Design review of the part built by this model. Coordinates are the model's own, in mm. A direction names the side the tool comes from. Coordinates: 2 decimals unless noted, no trailing zeros. Write each loop counter-clockwise with the first axis right and the second up, starting at its lowest first coordinate (ties: lowest second). Pieces come first, ordered by that corner, then holes.
Q1. Add section D-D, the plane z = -4.5. Give the boundary of the cut face in (x, y), plus the area to 3 significant figures.
Q2. Add section C-C, the plane y = 14. Give the boundary of the cut face in (x, z).
Q3. The part is to be moulded in two halves that separate along Y. For faces 1 (the face through (-3.905, 35.586, -0.867)), 2 (the face through (0, 36.6, 0)), 3 (the face through (0, 0, 0)), 4 (the face through (-1.141, 34.206, 3.625)), say which applies: +Y half, -Y half, draft (parallel to the pull), parting line (faces both ways), or undercut.
Q4. Machinability: for faces 5 (the face through (-4.88, 0.99, -1.08)), 6 (the face through (-3.905, 17.677, -0.867)), which of the approach directions +Z, -Z, +X, -X, +Y, -Y give a long, thin tool a straight path to every point of the face, cutting with its end or side? Answer none if there is none.
Q5. Clearance check with flat-ended pins moving along their axes: pin 1 Ø4 at (y, z) = (9.5, -4) entering from -X; pin 2 Ø2 at (x, y) = (-3.5, 32.5) entering from -Z; pin 3 Ø4 at (y, z) = (31, 0) entering from +X. State where each tip first meets the part, or that it passes through.
Q6. To check wall thickness, follow probe 1 along Y at (x, z) = (-2.75, -2.75); probe 2 along Y at (x, z) = (4, -2.25); probe 3 along X at (y, z) = (21, -0.25). State the ranges of each line that lie inside material, in increasing order.
Q7. Add section B-B, the plane x = 0. Give the boundary of the cut face in (y, z).
Q8. Add section A-A, the plane z = 0. Give the boundary of the cut face in (x, y), plus the area to 3 significant figures.
from build123d import *

# Parameters (mm, degrees)
SKETCH_1_R      = 5
EXTRUDE_1_DEPTH = 2
SKETCH_2_R      = 4
EXTRUDE_2_DEPTH = 34.6
SKETCH_3_W      = 0.4
SKETCH_3_H      = 0.8


with BuildPart() as part:
    # 草图1 → 凸台-拉伸1 (new body)
    with BuildSketch(Plane(origin=(0, 0, 0), x_dir=(1, 0, 0), z_dir=(0, 1, 0))):
        with Locations(Location((0, 0, 0), (0, 0, 270))):
            Circle(SKETCH_1_R)
    extrude(amount=EXTRUDE_1_DEPTH)

    # 草图2 → 凸台-拉伸2 (add)
    with BuildSketch(Plane(origin=(0, 2, 0), x_dir=(1, 0, 0), z_dir=(0, 1, 0))):
        with Locations(Location((0, 0, 0), (0, 0, 270))):
            Circle(SKETCH_2_R)
    extrude(amount=EXTRUDE_2_DEPTH)

    # 草图3 → 切除-旋转1 (revolve, cut)
    with BuildSketch(Plane.XY, mode=Mode.PRIVATE) as cut_revolve_1_sk:
        with Locations((4, 34.2)):
            Rectangle(SKETCH_3_W, SKETCH_3_H)
    revolve(cut_revolve_1_sk.sketch.rotate(Axis((0, 36.6, 0), (0, -1, 0)), 90), axis=Axis((0, 36.6, 0), (0, -1, 0)), mode=Mode.SUBTRACT)


solid = part.part
Here are the results:
1. outline: (-2.18, 0) - (2.18, 0) - (2.18, 2) - (-2.18, 2) - close
1. area: 8.72 mm2
2. outline: circle Ø8 at (0, 0)
3. face 1: draft
3. face 2: +Y half
3. face 3: -Y half
3. face 4: undercut
4. face 5: +Y, -Y
4. face 6: +Y
5. pin 1: stops at x = -3.46
5. pin 2: stops at z = -3.12
5. pin 3: stops at x = 4
6. probe 1: y = 0 to 33.8, 34.6 to 36.6
6. probe 2: y = 0 to 2
6. probe 3: x = -3.99 to 3.99
7. outline: (0, -5) - (2, -5) - (2, -4) - (33.8, -4) - (33.8, -3.8) - (34.6, -3.8) - (34.6, -4) - (36.6, -4) - (36.6, 4) - (34.6, 4) - (34.6, 3.8) - (33.8, 3.8) - (33.8, 4) - (2, 4) - (2, 5) - (0, 5) - close
8. outline: (-5, 0) - (5, 0) - (5, 2) - (4, 2) - (4, 33.8) - (3.8, 33.8) - (3.8, 34.6) - (4, 34.6) - (4, 36.6) - (-4, 36.6) - (-4, 34.6) - (-3.8, 34.6) - (-3.8, 33.8) - (-4, 33.8) - (-4, 2) - (-5, 2) - close
8. area: 296 mm2
